```python
from build123d import *

# Parameters (mm, degrees)
SKETCH1_W            = 157.864
SKETCH1_H            = 90.551
BOSS_EXTRUDE1_DEPTH  = 8
CUT_EXTRUDE21_DEPTH  = 5
FILLET8_R            = 2.75
SKETCH29_W           = 12.37533
SKETCH29_H           = 90.551
CUT_EXTRUDE25_DEPTH  = 183.166204596
FILLET9_R            = 5
SKETCH36_W           = 10
SKETCH36_H           = 10
SKETCH36_R           = 3.3
BOSS_EXTRUDE10_DEPTH = 8
FILLET10_R           = 2.5


with BuildPart() as part:
    # Sketch1 → Boss-Extrude1 (new body)
    with BuildSketch(Plane(origin=(0, 0, 0), x_dir=(1, 0, 0), z_dir=(0, 1, 0))):
        with Locations((78.932, -45.2755)):
            Rectangle(SKETCH1_W, SKETCH1_H)
    extrude(amount=BOSS_EXTRUDE1_DEPTH)

    # Sketch23 → Cut-Extrude21 (cut)
    with BuildSketch(Plane(origin=(0, 8, 0), x_dir=(1, 0, 0), z_dir=(0, 1, 0))):
        Polygon((141.332, -86.4755), (23.3181173, -86.4755), (16.532, -79.6893827), (16.532, -10.8616173), (23.3181173, -4.0755), (141.332, -4.0755), align=None)
    extrude(amount=-CUT_EXTRUDE21_DEPTH, mode=Mode.SUBTRACT)

    # Fillet8
    fillet8_edges = [part.edges().sort_by_distance(p)[0] for p in [
        (141.332, 5.5, 4.0755),
        (141.332, 5.5, 86.4755),
        (23.3181173, 5.5, 86.4755),
        (16.532, 5.5, 79.6893827),
        (16.532, 5.5, 10.8616173),
        (23.3181173, 5.5, 4.0755),
    ]]
    fillet(fillet8_edges, radius=FILLET8_R)

    # Sketch29 → Cut-Extrude25 (cut, through all)
    with BuildSketch(Plane(origin=(0, 8, 0), x_dir=(1, 0, 0), z_dir=(0, 1, 0))):
        with Locations((151.676335, -45.2755)):
            Rectangle(SKETCH29_W, SKETCH29_H)
        with Locations((6.187665, -45.2755)):
            Rectangle(SKETCH29_W, SKETCH29_H)
    extrude(amount=-CUT_EXTRUDE25_DEPTH, mode=Mode.SUBTRACT)

    # Fillet9
    fillet9_edges = [part.edges().sort_by_distance(p)[0] for p in [
        (145.48867, 4, 90.551),
        (145.48867, 4, 0),
        (12.37533, 4, 0),
        (12.37533, 4, 90.551),
    ]]
    fillet(fillet9_edges, radius=FILLET9_R)

    # Sketch36 → Boss-Extrude10 (add)
    # profile 1 of 4: a face of its own
    with BuildSketch(Plane.XZ):
        with Locations((26.3936, 95.551)):
            Rectangle(SKETCH36_W, SKETCH36_H)
        with Locations(Location((26.3936, 95.551, 0), (0, 0, 270))):
            Circle(SKETCH36_R, mode=Mode.SUBTRACT)
    # profile 2 of 4: a face of its own
    with BuildSketch(Plane.XZ):
        with Locations((129.6936, 95.551)):
            Rectangle(SKETCH36_W, SKETCH36_H)
        with Locations(Location((129.6936, 95.551, 0), (0, 0, 270))):
            Circle(SKETCH36_R, mode=Mode.SUBTRACT)
    # profile 3 of 4: a face of its own
    with BuildSketch(Plane.XZ):
        with Locations((26.3936, -5)):
            Rectangle(SKETCH36_W, SKETCH36_H)
        with Locations(Location((26.3936, -5, 0), (0, 0, 270))):
            Circle(SKETCH36_R, mode=Mode.SUBTRACT)
    # profile 4 of 4: a face of its own
    with BuildSketch(Plane.XZ):
        with Locations((129.6936, -5)):
            Rectangle(SKETCH36_W, SKETCH36_H)
        with Locations(Location((129.6936, -5, 0), (0, 0, 270))):
            Circle(SKETCH36_R, mode=Mode.SUBTRACT)
    extrude(amount=-BOSS_EXTRUDE10_DEPTH)

    # Fillet10
    fillet10_edges = [part.edges().sort_by_distance(p)[0] for p in [
        (21.3936, 4, 90.551),
        (21.3936, 4, 100.551),
        (31.3936, 4, 100.551),
        (31.3936, 4, 90.551),
        (124.6936, 4, 90.551),
        (124.6936, 4, 100.551),
        (134.6936, 4, 100.551),
        (134.6936, 4, 90.551),
        (31.3936, 4, 0),
        (31.3936, 4, -10),
        (21.3936, 4, -10),
        (21.3936, 4, 0),
        (124.6936, 4, -10),
        (124.6936, 4, 0),
        (134.6936, 4, 0),
        (134.6936, 4, -10),
    ]]
    fillet(fillet10_edges, radius=FILLET10_R)


solid = part.part
```
For this review, take the finished solid that the model builds, in its own axes (mm). A direction names the side the tool comes from. Coordinates: 2 decimals unless noted, no trailing zeros. Write each loop counter-clockwise with the first axis right and the second up, starting at its lowest first coordinate (ties: lowest second). Pieces come first, ordered by that corner, then holes.
(1) Add section A-A on z = -5. Give the boundary of the cut face in (x, y).
(2) The part is to be moulded in two halves that separate along Z. For faces 5 (the face through (19.96, 5.54, 83.12)), 6 (the face through (144.06, 3.94, 89.05)), 7 (the face through (140.548, 5.465, 4.902)), 8 (the face through (13.801, 3.944, 1.504)), say which applies: +Z half, -Z half, draft (parallel to the pull), parting line (faces both ways), or undercut.
(3) Tool access review of faces 1 (the face through (134.694, 4, -5)), 2 (the face through (19.889, 5.535, 7.505)), 3 (the face through (124.694, 4, -5)), 4 (the face through (77, 4, 90.551)): name each direction out of +Z, -Z, +X, -X, +Y, -Y from which nothing blocks a thin tool from reaching the whole face with its end or side.
(4) Wall thickness on probe 1 along X at (y, z) = (5, -5); probe 2 along Z at (x, y) = (91, 7); probe 3 along X at (y, z) = (6.75, 76): over which ranges is each line inside the solid? List them lowest first.
(5) Add section C-C on z = 32. Give the boundary of the cut face in (x, y), then the cut area to 3 significant figures.
(6) Add section B-B on x = 46.5. Give the boundary of the cut face in (y, z).
(7) For pin 1 Ø1.5 at (x, z) = (88.5, 87.5) entering from -Y; pin 2 Ø4 at (y, z) = (4.5, 95) entering from +X; pin 3 Ø1 at (x, y) = (88, 5.5) entering from -Z; pin 4 Ø3 at (x, y) = (86, 2) entering from +Z, all flat-tipped, find the tip position at first contact; note any pin that passes through.
Answer sheet:
1. outline: (21.39, 0) - (23.09, 0) - (23.09, 8) - (21.39, 8) - close; (29.69, 0) - (31.39, 0) - (31.39, 8) - (29.69, 8) - close; (124.69, 0) - (126.39, 0) - (126.39, 8) - (124.69, 8) - close; (132.99, 0) - (134.69, 0) - (134.69, 8) - (132.99, 8) - close
2. face 5: undercut
2. face 6: +Z half
2. face 7: undercut
2. face 8: -Z half
3. face 1: -Z, +X, +Y, -Y
3. face 2: +Y
3. face 3: -Z, +Y, -Y
3. face 4: +Z, +Y, -Y
4. probe 1: x = 21.39 to 23.09, 29.69 to 31.39, 124.69 to 126.39, 132.99 to 134.69
4. probe 2: z = 0 to 4.08, 86.48 to 90.55
4. probe 3: x = 12.38 to 16.53, 141.33 to 145.49
5. outline: (12.38, 0) - (145.49, 0) - (145.49, 8) - (141.33, 8) - (141.33, 3) - (16.53, 3) - (16.53, 8) - (12.38, 8) - close
5. area: 441 mm2
6. outline: (0, 0) - (8, 0) - (8, 4.08) - (3, 4.08) - (3, 86.48) - (8, 86.48) - (8, 90.55) - (0, 90.55) - close
7. pin 1: stops at y = 0
7. pin 2: stops at x = 134.69
7. pin 3: stops at z = 0
7. pin 4: stops at z = 90.55
